For this review, take the finished solid that the model builds, in its own axes (mm). A direction names the side the tool comes from. Coordinates: 2 decimals unless noted, no trailing zeros. Loops run counter-clockwise (first coordinate to the right, second up) from the corner with the lowest first, then second, coordinate; pieces in that order, holes last. Notation, with made-up numbers: (-22.5, 35.5) - (26.5, 35.5) arc R35 ccw to (26.5, 74.5) - close; hole circle Ø5 at (-5.75, 45.5). An arc over 180 degrees is marked (long way). Answer as a JSON object with one key per item and string values. Group by question number.
Item 1: To check wall thickness, follow line 1 (Z direction, x = 0, y = 9.75); line 2 (Y direction, x = -5, z = -8.5); line 3 (X direction, y = 6, z = 0.5). State the ranges of each line that lie inside material, in increasing order.
Item 2: Mouldability with a two-part tool opening along X and no side actions: class faces 6 (the cylindrical face through (34.003, -2.465, -40.253)), 7 (the flat face through (19, -2, -19)), 8 (the flat face through (15.79, -2.46, -20.1)), 9 (the flat face through (-8, 0, -12)) as released by +X, released by -X, zero draft, split by the parting line, or undercut.
Item 3: We need section B-B (y = 13.25). Give the boundary of the cut face in (x, z).
Item 4: We need section C-C (x = -3). Give the boundary of the cut face in (y, z).
Item 5: We need section D-D (y = 17.25). Give the boundary of the cut face in (x, z).
Item 6: We need section A-A (z = -33). Give the boundary of the cut face in (x, y), then the cut area to 3 significant figures.
Item 7: Clearance check with flat-ended pins moving along their axes: pin 1 (0.8 mm diameter, centred on x = 0.5, y = 16.5, fed in from +Z); pin 2 (5 mm diameter, centred on y = 9, z = -6, fed in from -X); pin 3 (2 mm diameter, centred on x = 0, y = 17.5, fed in from -Z). State where each tip first meets the part, or that it passes through.
Item 8: Tool access review of faces 1 (the flat face through (34.32, -2.46, -43.46)), 2 (the cylindrical face through (-36.82, -2.54, -38.84)), 3 (the flat face through (-16.23, -2.46, -20.54)), 4 (the cylindrical face through (-34.02, -2.46, -40.44)), 5 (the flat face through (0, 15, -2)): name each direction out of +Z, -Z, +X, -X, +Y, -Y from which nothing blocks a thin tool from reaching the whole face with its end or side.
from build123d import *
from build123d import SkipClean  # not in build123d's __all__

# Parameters (mm, degrees)
F1_DEPTH    = 5
F2_DEPTH    = 20
F3_R        = 5
F4_START    = -15
F4_DEPTH    = 5
F5_T1_DEPTH = 5


# Not quite as in the source:
# - a fillet or chamfer that OpenCascade refuses, or shapes differently, is made with other operations: its cross-section is extruded or revolved along the edge and cut away or added
# - after a boolean that leaves OpenCascade's solid faulty, fix() repairs it
# - a feature names something its author has since deleted; it is built from what else it names


with BuildPart() as f1:
    # F0 (on Front) → F1 (new body)
    with BuildSketch(Plane.XZ):
        with BuildLine():
            Line((0.0300982685, -4.2060010783), (-2.0879514049, -2.0879514049))
            Line((-2.0879514049, -2.0879514049), (-38.8908729653, -38.8908729653))
            Line((-38.8908729653, -38.8908729653), (-33.3183881591, -44.4633577714))
            Line((-33.3183881591, -44.4633577714), (-33.1233781652, -44.7987950851))
            ThreePointArc((-33.1233781652, -44.7987950851), (-34.0132139837, -40.3773459148), (-32.0214836094, -36.3308621737))
            Line((-32.0214836094, -36.3308621737), (0, -4.3093785644))
            Line((0, -4.3093785644), (0.0667378772, -4.2426406871))
            Line((0.0667378772, -4.2426406871), (0.0300982685, -4.2060010783))
        make_face()
        with BuildLine():
            Line((-4.1759028099, 0), (-2.0879514049, -2.0879514049))
            Line((-2.0879514049, -2.0879514049), (-1.8201223283, -1.8201223283))
            ThreePointArc((-1.8201223283, -1.8201223283), (-0.6954224476, 1.6424563629), (2.25, -0.4973771865))
            ThreePointArc((2.25, -0.4973771865), (2.1398335494, -1.1927996342), (1.8201223283, -1.8201223283))
            Line((1.8201223283, -1.8201223283), (2.1546892822, -2.1546892822))
            Line((2.1546892822, -2.1546892822), (2.2214271594, -2.0879514049))
            Line((2.2214271594, -2.0879514049), (4.3093785644, 0))
            Line((4.3093785644, 0), (0.0333689386, 4.2092717485))
            Line((0.0333689386, 4.2092717485), (-4.1759028099, 0))
        make_face()
        with BuildLine():
            Line((-1.8201223283, -1.8201223283), (-2.0879514049, -2.0879514049))
            Line((-2.0879514049, -2.0879514049), (0.0300982685, -4.2060010783))
            Line((0.0300982685, -4.2060010783), (0.0667378772, -4.2426406871))
            Line((0.0667378772, -4.2426406871), (2.1546892822, -2.1546892822))
            Line((2.1546892822, -2.1546892822), (1.8201223283, -1.8201223283))
            ThreePointArc((1.8201223283, -1.8201223283), (0, -2.7473771865), (-1.8201223283, -1.8201223283))
        make_face()
        Polygon((2.1546892822, -2.1546892822), (0.0667378772, -4.2426406871), (0, -4.3093785644), (35.8313777613, -40.1407563256), (33.3183881591, -44.4633577714), (38.8908729653, -38.8908729653), align=None)
    extrude(amount=F1_DEPTH)

    # F0 (on Front) → F2 (join)
    with BuildSketch(Plane.XZ):
        with BuildLine():
            Line((-4.1759028099, 0), (-2.0879514049, -2.0879514049))
            Line((-2.0879514049, -2.0879514049), (-1.8201223283, -1.8201223283))
            ThreePointArc((-1.8201223283, -1.8201223283), (-0.6954224476, 1.6424563629), (2.25, -0.4973771865))
            ThreePointArc((2.25, -0.4973771865), (2.1398335494, -1.1927996342), (1.8201223283, -1.8201223283))
            Line((1.8201223283, -1.8201223283), (2.1546892822, -2.1546892822))
            Line((2.1546892822, -2.1546892822), (2.2214271594, -2.0879514049))
            Line((2.2214271594, -2.0879514049), (4.3093785644, 0))
            Line((4.3093785644, 0), (0.0333689386, 4.2092717485))
            Line((0.0333689386, 4.2092717485), (-4.1759028099, 0))
        make_face()
        with BuildLine():
            Line((-1.8201223283, -1.8201223283), (-2.0879514049, -2.0879514049))
            Line((-2.0879514049, -2.0879514049), (0.0300982685, -4.2060010783))
            Line((0.0300982685, -4.2060010783), (0.0667378772, -4.2426406871))
            Line((0.0667378772, -4.2426406871), (2.1546892822, -2.1546892822))
            Line((2.1546892822, -2.1546892822), (1.8201223283, -1.8201223283))
            ThreePointArc((1.8201223283, -1.8201223283), (0, -2.7473771865), (-1.8201223283, -1.8201223283))
        make_face()
    with SkipClean():  # cleaning this boolean's faces spoils the solid; the shape is the same uncleaned
        extrude(amount=-F2_DEPTH)

    # F3
    f3_edges = [f1.edges().sort_by_distance(p)[0] for p in [
        (38.890873, -2.5, -38.890873),
        (-38.890873, -2.5, -38.890873),
    ]]
    fillet(f3_edges, radius=F3_R)

    # F0 (on Front) → F4 (join)
    with BuildSketch(Plane.XZ.offset(F4_START)):
        with BuildLine():
            Line((1.2727922061, -1.2727922061), (1.4969489762, -1.4969489762))
            ThreePointArc((1.4969489762, -1.4969489762), (1.7225719371, -1.0196280089), (1.8, -0.4973771865))
            ThreePointArc((1.8, -0.4973771865), (1.6629831585, 0.1914529917), (1.2727922061, 0.7754150196))
            Line((1.2727922061, 0.7754150196), (1.2727922061, -1.2727922061))
        make_face()
        with BuildLine():
            ThreePointArc((1.2727922061, -1.7701693927), (1.3915922187, -1.6390737735), (1.4969489762, -1.4969489762))
            Line((1.4969489762, -1.4969489762), (1.2727922061, -1.2727922061))
            Line((1.2727922061, -1.2727922061), (1.2727922061, -1.7701693927))
        make_face()
        with BuildLine():
            Line((-1.2727922061, -1.2727922061), (-1.4969489762, -1.4969489762))
            ThreePointArc((-1.4969489762, -1.4969489762), (-1.3915922187, -1.6390737735), (-1.2727922061, -1.7701693927))
            Line((-1.2727922061, -1.7701693927), (-1.2727922061, -1.2727922061))
        make_face()
        with BuildLine():
            Line((1.2727922061, -1.7701693927), (-1.2727922061, -1.7701693927))
            ThreePointArc((-1.2727922061, -1.7701693927), (0, -2.2973771865), (1.2727922061, -1.7701693927))
        make_face()
        with BuildLine():
            ThreePointArc((-1.2727922061, 0.7754150196), (-1.7913056932, -0.3206742907), (-1.4969489762, -1.4969489762))
            Line((-1.4969489762, -1.4969489762), (-1.2727922061, -1.2727922061))
            Line((-1.2727922061, -1.2727922061), (-1.2727922061, 0.7754150196))
        make_face()
        with BuildLine():
            ThreePointArc((1.2727922061, 0.7754150196), (0, 1.3026228135), (-1.2727922061, 0.7754150196))
            Line((-1.2727922061, 0.7754150196), (1.2727922061, 0.7754150196))
        make_face()
        with BuildLine():
            ThreePointArc((2.25, -0.4973771865), (-0.6954224476, 1.6424563629), (-1.8201223283, -1.8201223283))
            Line((-1.8201223283, -1.8201223283), (-1.4969489762, -1.4969489762))
            ThreePointArc((-1.4969489762, -1.4969489762), (-1.7913056932, -0.3206742907), (-1.2727922061, 0.7754150196))
            ThreePointArc((-1.2727922061, 0.7754150196), (0, 1.3026228135), (1.2727922061, 0.7754150196))
            ThreePointArc((1.2727922061, 0.7754150196), (1.6629831585, 0.1914529917), (1.8, -0.4973771865))
            ThreePointArc((1.8, -0.4973771865), (1.7225719371, -1.0196280089), (1.4969489762, -1.4969489762))
            Line((1.4969489762, -1.4969489762), (1.8201223283, -1.8201223283))
            ThreePointArc((1.8201223283, -1.8201223283), (2.1398335494, -1.1927996342), (2.25, -0.4973771865))
        make_face()
        with BuildLine():
            Line((-1.4969489762, -1.4969489762), (-1.8201223283, -1.8201223283))
            ThreePointArc((-1.8201223283, -1.8201223283), (0, -2.7473771865), (1.8201223283, -1.8201223283))
            Line((1.8201223283, -1.8201223283), (1.4969489762, -1.4969489762))
            ThreePointArc((1.4969489762, -1.4969489762), (1.3915922187, -1.6390737735), (1.2727922061, -1.7701693927))
            ThreePointArc((1.2727922061, -1.7701693927), (0, -2.2973771865), (-1.2727922061, -1.7701693927))
            ThreePointArc((-1.2727922061, -1.7701693927), (-1.3915922187, -1.6390737735), (-1.4969489762, -1.4969489762))
        make_face()
    extrude(amount=-F4_DEPTH)

    add(f1.part.fix(), mode=Mode.REPLACE)

    # F5: fillet of radius 7 on 1 edges, made by hand

    # F5_s2 → F5_t1 (join)
    with BuildSketch(Plane.XZ):
        with BuildLine():
            ThreePointArc((33.3183881591, -44.4633577714), (33.9932652456, -40.1917985218), (32.0294732352, -36.3388517995))
            Line((32.0294732352, -36.3388517995), (35.8313777613, -40.1407563256))
            Line((35.8313777613, -40.1407563256), (33.3183881591, -44.4633577714))
        make_face()
    extrude(amount=F5_T1_DEPTH)


solid = f1.part
Check sheet entries:
{
 "1": {"line 1": "z = -4.18 to -2.75, 1.75 to 4.18", "line 2": "y = -5 to 0", "line 3": "x = -3.68 to -2.02, 2.02 to 3.8"},
 "2": {"face 6": "undercut", "face 7": "released by +X", "face 8": "undercut", "face 9": "zero draft"},
 "3": {"outline": "(-4.18, 0) - (0.07, -4.24) - (4.31, 0) - (0.03, 4.21) - close; hole circle Ø4.5 at (0, -0.5)"},
 "4": {"outline": "(-5, -7.31) - (0, -7.31) - (0, -3) - (-5, -3) - close; (-5, -1.18) - (20, -1.18) - (20, 1.18) - (-5, 1.18) - close"},
 "5": {"outline": "(-4.18, 0) - (0.07, -4.24) - (4.31, 0) - (0.03, 4.21) - close; hole (-1.27, -1.77) - (1.27, -1.77) - (1.27, 0.78) - (-1.27, 0.78) - close"},
 "6": {"outline": "(-33, -5) - (-28.69, -5) - (-28.69, 0) - (-33, 0) - close; (28.69, -5) - (33, -5) - (33, 0) - (28.69, 0) - close", "area": "43.1 mm2"},
 "7": {"pin 1": "stops at z = 4.14", "pin 2": "stops at x = -0.68", "pin 3": "stops at z = -4.24"},
 "8": {"face 1": "-Z, +X, +Y, -Y", "face 2": "-X, +Y, -Y", "face 3": "-Z, +Y, -Y", "face 4": "+Y, -Y", "face 5": "-Y"}
}
